Can you work these out from the model? Positions are in its coordinate system, mm. A direction names the side the tool comes from. Round coordinates to 2 decimals unless told otherwise and drop trailing zeros. Order: outer loops, then holes, each group sorted by start corner. A loop starts at its lowest first (then second) coordinate and runs counter-clockwise, first axis right, second up. Notation, with made-up numbers: M 48,23 L 86,23 A10 ccw 86,41 Z; hole C -12.75,6 d4. An arc over 180 degrees is marked long. One line per question, with ' | ' between items.
```python
from build123d import *

# Parameters (mm, degrees)
F1_DEPTH = 7.5
F3_D     = 20
F5_D     = 4.2
F7_D     = 11


with BuildPart() as f1:
    # F0 (on Front) → F1 (new body, symmetric)
    with BuildSketch(Plane.XZ):
        Polygon((-300, 222), (-300, -290), (300, -290), (300, 222), (130, 222), (130, 0), (-74, 0), (-74, 138), (-20, 192), (-20, 222), align=None)
    extrude(amount=F1_DEPTH, both=True)

    # F3 (through all)
    with Locations(Plane(origin=(0, 7.5, 0), x_dir=(-1, 0, 0), z_dir=(0, 1, 0))):
        with Locations((-245, 196), (205, 196), (-245, -4), (205, -4)):
            Hole(F3_D / 2)

    # F5 (through all)
    with Locations(Plane(origin=(0, 7.5, 0), x_dir=(-1, 0, 0), z_dir=(0, 1, 0))):
        with Locations((-210.69, -117.89), (-234.73, -93.85), (-149.39, -25.55), (155.66, -152.66), (223.96, -248), (251, -220.96), (95.42, 135.79), (121.9, 162.27)):
            Hole(F5_D / 2)

    # F7 (through all)
    with Locations(Plane(origin=(0, 7.5, 0), x_dir=(-1, 0, 0), z_dir=(0, 1, 0))):
        with Locations((-277, 196), (-277, -4), (237, 196), (237, -4)):
            Hole(F7_D / 2)


solid = f1.part
```
(1) If we section it at B-B on y = -4.75: State how many separate pieces and enclosed holes the cut face has, plus the area to 3 significant figures.
Final values:
separate pieces: 1 | enclosed holes: 16 | area: 263,000 mm^2
(2) If we section it at D-D on z = 153: Please give me the cut outline in (x, y), plus the area to 4 significant figures.
Final values:
outline: M -300,-7.5 L -59,-7.5 L -59,7.5 L -300,7.5 Z; M 130,-7.5 L 300,-7.5 L 300,7.5 L 130,7.5 Z | area: 6,165 mm^2
(3) On a 3-axis mill with a long thin cutter (end or side, diameter ignored), from which of +Z, -Z, +X, -X, +Y, -Y can I reach the whole of each face in a straight line? I mean faces 1 (the flat face through (-20, 0, 207)), 2 (the flat face through (-4, 0, -290)), 3 (the flat face through (29, 0, 0)). Say none if no direction works.
Final values:
face 1: +Z, +Y, -Y | face 2: -Z, +X, -X, +Y, -Y | face 3: +Y, -Y
(4) If we section it at A-A on z = 54.5: Please give me the cut outline in (x, y), plus the area to 3 significant figures.
Final values:
outline: M -300,-7.5 L -74,-7.5 L -74,7.5 L -300,7.5 Z; M 130,-7.5 L 300,-7.5 L 300,7.5 L 130,7.5 Z | area: 5,940 mm^2
(5) Will these pins go through, and if not, where does the flat tip stop? pin 1 Ø6.5 at (x, z) = (277, 196) entering from -Y; pin 2 Ø5.5 at (x, z) = (210.69, -117.89) entering from -Y.
Final values:
pin 1: through | pin 2: y = -7.5
(6) Please list where these lines run through material, in increasing order: probe 1 along Z at (x, y) = (245, -0.75); probe 2 along Z at (x, y) = (-237, 0); probe 3 along Z at (x, y) = (-223.96, -0.75). Write a range as [from, to].
Final values:
probe 1: [-290, -14], [6, 186], [206, 222] | probe 2: [-290, -9.5], [1.5, 190.5], [201.5, 222] | probe 3: [-290, -250.1], [-245.9, 222]
(7) Thinking about a two-plate mould opening in X: for faces 4 (the flat face through (130, 0, 113)), 5 (the flat face through (-300, 0, -30)), 6 (the flat face through (-4, 7.5, -87)), which applies, released by +X, released by -X, zero draft, split by the parting line, or undercut?
Final values:
face 4: undercut | face 5: released by -X | face 6: zero draft
(8) If we section it at C-C on x = 27: Please give me the cut outline in (y, z).
Final values:
outline: M -7.5,-290 L 7.5,-290 L 7.5,0 L -7.5,0 Z
